Geometry: final body of the model. Coordinates: model frame, mm. A direction names the side the tool comes from. Give positions to 0.01 mm unless a question says otherwise; leave off trailing zeros. Write each loop counter-clockwise with the first axis right and the second up, starting at its lowest first coordinate (ties: lowest second). Pieces come first, ordered by that corner, then holes.
Q1. Mould query, pull axis X, two halves, no side actions, for faces 4 (the flat face through (7.366, 33, 7)), 5 (the cylindrical face through (34.73, 10.92, 0.79)), 6 (the flat face through (74, 3.048, 7)), 7 (the flat face through (7.112, 33, 7)). Classes: +X half, -X half, draft (parallel to the pull), parting line (faces both ways), or undercut.
Q2. Reachability of faces 1 (the flat face through (76, 18, 0)), 2 (the flat face through (74, 64.516, 7)), 3 (the flat face through (142.748, 33, 7)) from +Z, -Z, +X, -X, +Y, -Y: full face, straight path, thin tool, end or side. Return the list, or none.
Q3. Line query: line 1 (X direction, y = 56.5, z = 5); line 2 (Y direction, x = 141.5, z = 12); line 3 (Z direction, x = 94, y = 63). Output: solid intervals per line, ascending.
Q4. Section A-A (x = 92). Return the cut outline in (y, z).
Q5. Section B-B (y = 42.5). Return the cut outline in (x, z).
Q6. Section C-C (z = 10.5). Return the cut outline in (x, y).
Q7. Pin query (flat end, axial travel): pin 1 Ø4 at (x, y) = (108, 15.5) entering from +Z; pin 2 Ø2.5 at (x, y) = (139.24, 61.57) entering from -Z; pin 3 Ø1 at (y, z) = (6.5, 7.5) entering from +X; pin 4 Ø4 at (x, z) = (47, 4.5) entering from -Y. Return the tip coordinate at first contact, or that it passes through.
from build123d import *

# Parameters (mm, degrees)
BOSS_EXTRUDE1_DEPTH  = 1.6002
CUT_EXTRUDE1_DEPTH   = 169.893706928
CUT_EXTRUDE2_DEPTH   = 169.893706928
CUT_EXTRUDE3_DEPTH   = 169.893706928
CUT_EXTRUDE4_DEPTH   = 169.893706928
SKETCH6_W            = 135.636
SKETCH6_H            = 61.722
BOSS_EXTRUDE2_DEPTH  = 11
SKETCH7_W            = 135.128
SKETCH7_H            = 61.214
CUT_EXTRUDE5_DEPTH   = 11
SKETCH8_W            = 75.184
SKETCH8_H            = 24.384
CUT_EXTRUDE6_DEPTH   = 170.243976555
SKETCH9_W            = 11.792676588
SKETCH9_H            = 1.790289347
CUT_EXTRUDE7_DEPTH   = 170.355509624
M2_CLEARANCE_HOLE1_D = 2.39776
M4_CLEARANCE_HOLE1_D = 4.445
M4_CLEARANCE_HOLE2_D = 4.68589235


with BuildPart() as part:
    # Sketch1 → Boss-Extrude1 (new body)
    with BuildSketch(Plane.XY.offset(1.6002)):
        Polygon((6.35, 70.612), (0, 64.262), (0, 3.81), (6.35, -2.54), (147.066, -2.54), (153.416, 3.81), (153.416, 64.262), (147.066, 70.612), align=None)
    extrude(amount=-BOSS_EXTRUDE1_DEPTH)

    # Sketch2 → Cut-Extrude1 (cut, through all)
    with BuildSketch(Plane(origin=(0, 0, 0), x_dir=(-1, 0, 0), z_dir=(0, 0, -1))):
        with BuildLine():
            Line((-153.416, 9.525), (-153.416, 5.715))
            Line((-153.416, 5.715), (-149.606, 5.715))
            ThreePointArc((-149.606, 5.715), (-147.701, 7.62), (-149.606, 9.525))
            Line((-149.606, 9.525), (-153.416, 9.525))
        make_face()
    extrude(amount=-CUT_EXTRUDE1_DEPTH, mode=Mode.SUBTRACT)

    # Sketch3 → Cut-Extrude2 (cut, through all)
    with BuildSketch(Plane(origin=(0, 0, 0), x_dir=(-1, 0, 0), z_dir=(0, 0, -1))):
        with BuildLine():
            Line((-153.416, 62.357), (-153.416, 58.547))
            Line((-153.416, 58.547), (-149.606, 58.547))
            ThreePointArc((-149.606, 58.547), (-147.701, 60.452), (-149.606, 62.357))
            Line((-149.606, 62.357), (-153.416, 62.357))
        make_face()
    extrude(amount=-CUT_EXTRUDE2_DEPTH, mode=Mode.SUBTRACT)

    # Sketch4 → Cut-Extrude3 (cut, through all)
    with BuildSketch(Plane(origin=(0, 0, 0), x_dir=(-1, 0, 0), z_dir=(0, 0, -1))):
        with BuildLine():
            Line((0, 58.547), (0, 62.357))
            Line((0, 62.357), (-3.81, 62.357))
            ThreePointArc((-3.81, 62.357), (-5.715, 60.452), (-3.81, 58.547))
            Line((-3.81, 58.547), (0, 58.547))
        make_face()
    extrude(amount=-CUT_EXTRUDE3_DEPTH, mode=Mode.SUBTRACT)

    # Sketch5 → Cut-Extrude4 (cut, through all)
    with BuildSketch(Plane(origin=(0, 0, 0), x_dir=(-1, 0, 0), z_dir=(0, 0, -1))):
        with BuildLine():
            Line((0, 5.715), (0, 9.525))
            Line((0, 9.525), (-3.81, 9.525))
            ThreePointArc((-3.81, 9.525), (-5.715, 7.62), (-3.81, 5.715))
            Line((-3.81, 5.715), (0, 5.715))
        make_face()
    extrude(amount=-CUT_EXTRUDE4_DEPTH, mode=Mode.SUBTRACT)

    # Sketch6 → Boss-Extrude2 (add)
    with BuildSketch(Plane.XY.offset(1.6002)):
        with Locations((74.93, 33.909)):
            Rectangle(SKETCH6_W, SKETCH6_H)
    extrude(amount=BOSS_EXTRUDE2_DEPTH)

    # Sketch7 → Cut-Extrude5 (cut)
    with BuildSketch(Plane.XY.offset(12.6002)):
        with Locations((74.93, 33.909)):
            Rectangle(SKETCH7_W, SKETCH7_H)
    extrude(amount=-CUT_EXTRUDE5_DEPTH, mode=Mode.SUBTRACT)

    # Sketch8 → Cut-Extrude6 (cut, through all)
    with BuildSketch(Plane.XY.offset(1.6002)):
        with Locations((92.71, 34.036)):
            Rectangle(SKETCH8_W, SKETCH8_H)
    extrude(amount=-CUT_EXTRUDE6_DEPTH, mode=Mode.SUBTRACT)

    # Sketch9 → Cut-Extrude7 (cut, through all)
    with BuildSketch(Plane(origin=(0, 0, 0), x_dir=(-1, 0, 0), z_dir=(0, 0, -1))):
        with Locations((-17.905053156, 12.47860787)):
            Rectangle(SKETCH9_W, SKETCH9_H)
    extrude(amount=-CUT_EXTRUDE7_DEPTH, mode=Mode.SUBTRACT)

    # M2 Clearance Hole1 (through all)
    with Locations(Plane.XY.offset(1.6002)):
        with Locations((127.4445, 6.98246), (127.44958, 11.303), (57.4548, 7.03326), (57.43956, 11.32332)):
            Hole(M2_CLEARANCE_HOLE1_D / 2)

    # M4 Clearance Hole1 (through all)
    with Locations(Plane.XY.offset(1.6002)):
        with Locations((46.228, 61.5696), (46.228, 6.5786), (139.2174, 6.5786), (139.2428, 61.5696)):
            Hole(M4_CLEARANCE_HOLE1_D / 2)

    # M4 Clearance Hole2 (through all)
    with Locations(Plane.XY.offset(1.6002)):
        with Locations((34.22065157, 13.205568935)):
            Hole(M4_CLEARANCE_HOLE2_D / 2)


solid = part.part
Computed:
1. face 4: undercut
1. face 5: undercut
1. face 6: draft
1. face 7: -X half
2. face 1: -Z, +X, -X, +Y, -Y
2. face 2: +Z
2. face 3: +Z, +X, +Y, -Y
3. line 1: x = 7.11 to 7.37, 142.49 to 142.75
3. line 2: y = 3.05 to 3.3, 64.52 to 64.77
3. line 3: z = 0 to 1.6
4. outline: (-2.54, 0) - (21.84, 0) - (21.84, 1.6) - (3.3, 1.6) - (3.3, 12.6) - (3.05, 12.6) - (3.05, 1.6) - (-2.54, 1.6) - close; (46.23, 0) - (70.61, 0) - (70.61, 1.6) - (64.77, 1.6) - (64.77, 12.6) - (64.52, 12.6) - (64.52, 1.6) - (46.23, 1.6) - close
5. outline: (0, 0) - (55.12, 0) - (55.12, 1.6) - (7.37, 1.6) - (7.37, 12.6) - (7.11, 12.6) - (7.11, 1.6) - (0, 1.6) - close; (130.3, 0) - (153.42, 0) - (153.42, 1.6) - (142.75, 1.6) - (142.75, 12.6) - (142.49, 12.6) - (142.49, 1.6) - (130.3, 1.6) - close
6. outline: (7.11, 3.05) - (142.75, 3.05) - (142.75, 64.77) - (7.11, 64.77) - close; hole (7.37, 3.3) - (142.49, 3.3) - (142.49, 64.52) - (7.37, 64.52) - close
7. pin 1: stops at z = 1.6
7. pin 2: passes through
7. pin 3: stops at x = 142.75
7. pin 4: stops at y = 3.05
